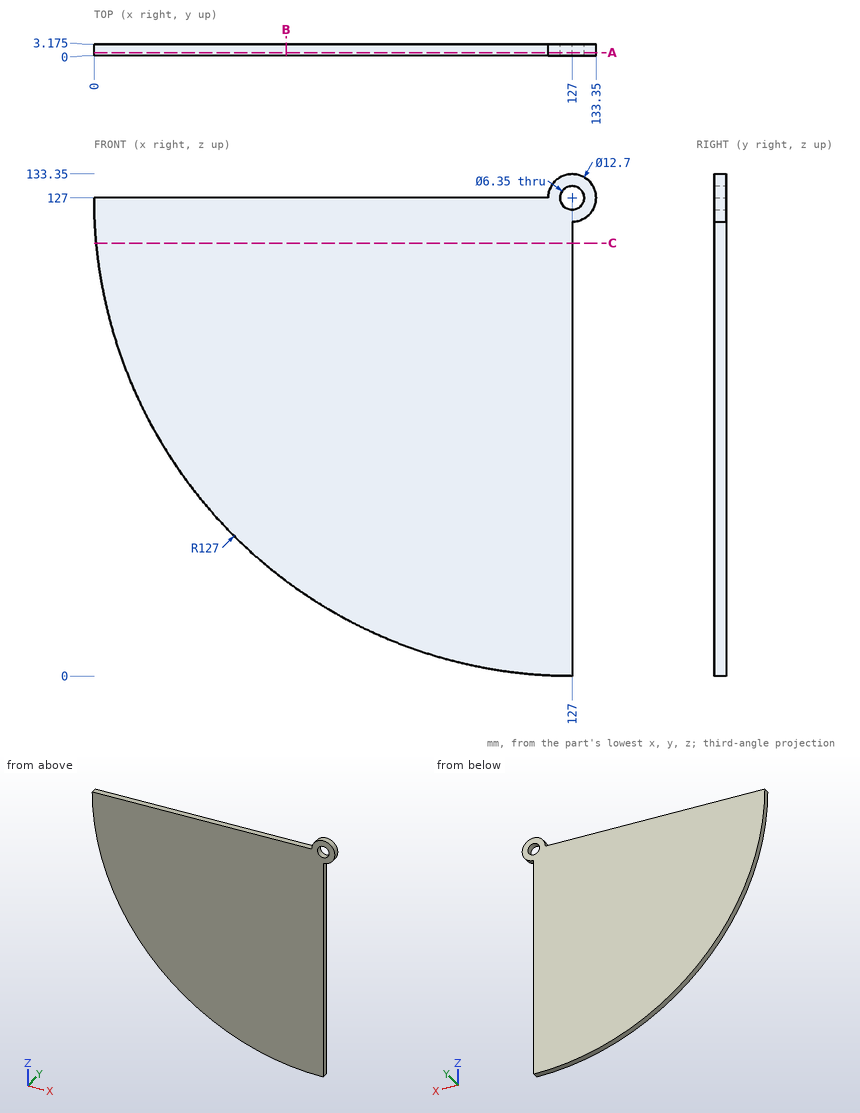
Can you work these out from the drawing? Everything is in mm from the part's minimum corner. Give positions to 0.01 mm unless a question says otherwise; leave off trailing zeros. Order: outer loops, then holes, each group sorted by start corner. A loop starts at its lowest first (then second) coordinate and runs counter-clockwise, first axis right, second up. Notation, with made-up numbers: (55.5, 22.25) -> (85.5, 22.25) arc R16 cw to (85.5, 53.25) -> close; hole circle Ø3 at (-29.5, 68). An arc over 180 degrees is marked (long way). Return JSON: item names as keys, results as strings.
1. Imagine slicing it at A-A on y = 0.9. List the corners of the cut face in (x, z) for me (3 decimals).
Answer list:
{"outline": "(0, 127) arc R127 ccw to (127, 0) -> (127, 120.65) arc R6.35 ccw (long way) to (120.65, 127) -> close; hole circle Ø6.35 at (127, 127)"}
2. Imagine slicing it at B-B on x = 51. List the corners of the cut face in (y, z) for me (3 decimals).
Answer list:
{"outline": "(0, 25.25) -> (3.175, 25.25) -> (3.175, 127) -> (0, 127) -> close"}
3. Imagine slicing it at C-C on z = 115. List the corners of the cut face in (x, y) for me (3 decimals).
Answer list:
{"outline": "(0.568, 0) -> (127, 0) -> (127, 3.175) -> (0.568, 3.175) -> close"}
4. I need wall thicknesses on line 1 (X direction, y = 2.35, z = 113.5); line 2 (Z direction, x = 24, y = 0.85); line 3 (X direction, y = 0.35, z = 117.5). Which ranges of each line are inside material? Lowest first, please. Write a range as from..to.
Answer list:
{"line 1": "x = 0.72..127", "line 2": "z = 52.7..127", "line 3": "x = 0.36..127"}
